```python
from build123d import *

# Parameters (mm, degrees)
SKETCH2_W           = 15.875
SKETCH2_H           = 3.175
BOSS_EXTRUDE1_DEPTH = 9.3472
SKETCH3_W           = 2.413
SKETCH3_H           = 9.525
CUT_EXTRUDE1_DEPTH  = 13.7
SKETCH4_R           = 1.45
BOSS_EXTRUDE2_DEPTH = 5.08


with BuildPart() as part:
    # Sketch2 → Boss-Extrude1 (new body)
    with BuildSketch(Plane(origin=(0, 0, 0), x_dir=(0, 0, -1), z_dir=(1, 0, 0))):
        with Locations((-7.9375, -1.5875)):
            Rectangle(SKETCH2_W, SKETCH2_H)
        Polygon((0, 9.525), (0, 0), (0, -3.175), (12.7, -3.175), (12.7, 9.525), align=None)
    extrude(amount=BOSS_EXTRUDE1_DEPTH)

    # Sketch3 → Cut-Extrude1 (cut, through all)
    with BuildSketch(Plane(origin=(0, 9.525, 0), x_dir=(1, 0, 0), z_dir=(0, 1, 0))):
        with Locations((4.6736, 7.9375)):
            Rectangle(SKETCH3_W, SKETCH3_H)
        Polygon((3.4671, 3.175), (3.4671, 12.7), (3.4036, 12.7), align=None)
        Polygon((5.9436, 12.7), (5.8801, 12.7), (5.8801, 3.175), align=None)
    extrude(amount=-CUT_EXTRUDE1_DEPTH, mode=Mode.SUBTRACT)

    # Sketch4 → Boss-Extrude2 (add)
    with BuildSketch(Plane.XZ.offset(3.175)):
        with Locations((4.6736, 12.7)):
            Circle(SKETCH4_R)
        with Locations((4.6736, 6.35)):
            Circle(SKETCH4_R)
    extrude(amount=BOSS_EXTRUDE2_DEPTH)


solid = part.part
```
Work out the finished part from the listing and answer in its coordinate system (mm). A direction names the side the tool comes from. Give positions to 0.01 mm unless a question says otherwise; leave off trailing zeros. Write each loop counter-clockwise with the first axis right and the second up, starting at its lowest first coordinate (ties: lowest second). Pieces come first, ordered by that corner, then holes. Notation, with made-up numbers: (45.5, 49) - (75.5, 49) arc R12 ccw to (75.5, 71) - close; hole circle Ø2 at (82, -4.5). An arc over 180 degrees is marked (long way). Use one line per item in the form item = value.
1. A cutting plane is placed at A-A (z = -9.5). Write down the section's boundary in (x, y) (3 decimals), and give its area (3 significant figures).
Filled in:
outline = (0, -3.175) - (3.425, -3.175) - (3.425, 9.525) - (0, 9.525) - close; (5.922, -3.175) - (9.347, -3.175) - (9.347, 9.525) - (5.922, 9.525) - close
area = 87.0 mm^2
2. Consider L1, parallel to Y at x = 7.5, z = 4.25 (3 decimals); L2, parallel to Y at x = 8.75, z = -10.5 (3 decimals); L3, parallel to Z at x = 8.5, y = 6.5. Determine where each line is inside the solid, lowest interval first.
Filled in:
L1 = -3.175 to 0
L2 = -3.175 to 9.525
L3 = -12.7 to 0
3. A cutting plane is placed at C-C (y = 3). Write down the section's boundary in (x, z) (3 decimals), and give its area (3 significant figures).
Filled in:
outline = (0, -12.7) - (3.404, -12.7) - (3.467, -3.175) - (5.88, -3.175) - (5.944, -12.7) - (9.347, -12.7) - (9.347, 0) - (0, 0) - close
area = 95.1 mm^2
4. Each of these flat-tipped pins is pushed along its axis until it touches: pin 1 Ø4.5 at (x, z) = (4, -5) entering from -Y (3 decimals); pin 2 Ø4.5 at (x, z) = (4.5, 5.5) entering from +Y; pin 3 Ø4.5 at (x, y) = (4, 2.5) entering from +Z. Where does it stop, or does it pass through?
Filled in:
pin_1 = -3.175
pin_2 = 0
pin_3 = 0
5. A cutting plane is placed at D-D (z = 12.7). Write down the section's boundary in (x, y) (3 decimals).
Filled in:
outline = (0, -3.175) - (3.224, -3.175) - (3.224, -8.255) - (6.124, -8.255) - (6.124, -3.175) - (9.347, -3.175) - (9.347, 0) - (0, 0) - close
6. Determine the mould class of faces 6 (the face through (5, 5, 0)), 7 (the face through (5.453, -5.679, 13.923)), 8 (the face through (8, 3, -12.7)) for opening direction Z: released by +Z, released by -Z, zero draft, split by the parting line, or undercut.
Filled in:
face_6 = released by +Z
face_7 = undercut
face_8 = released by -Z
7. A cutting plane is placed at B-B (x = 5). Write down the section's boundary in (y, z) (3 decimals).
Filled in:
outline = (-8.255, 4.937) - (-3.175, 4.937) - (-3.175, -3.175) - (9.525, -3.175) - (9.525, 0) - (0, 0) - (0, 15.875) - (-3.175, 15.875) - (-3.175, 14.113) - (-8.255, 14.113) - (-8.255, 11.287) - (-3.175, 11.287) - (-3.175, 7.763) - (-8.255, 7.763) - close
8. For faces 1 (the face through (5.34, -5.68, 5.06)), 2 (the face through (7, 9.525, -6)), 3 (the face through (0, 2, -5)), 4 (the face through (5, 3, -3.175)), 5 (the face through (5, 0, 8)), determine the directions among +Z, -Z, +X, -X, +Y, -Y from which every point of the face is accessible in a straight line to the end or side of a thin tool.
Filled in:
face_1 = -Y
face_2 = +Z, -Z, +X, -X, +Y
face_3 = +Z, -Z, -X, +Y, -Y
face_4 = -Z, +Y, -Y
face_5 = +Z, +X, -X, +Y
